```python
from build123d import *

# Parameters (mm, degrees)
SKETCH_1_R      = 7.5
SKETCH_1_R_2    = 2.7
EXTRUDE_1_DEPTH = 3
SKETCH_3_R      = 4
SKETCH_3_R_2    = 2.7
EXTRUDE_3_DEPTH = 32.5
EXTRUDE_START   = -32.5
SKETCH_4_R      = 6
SKETCH_4_R_2    = 2.7
EXTRUDE_4_DEPTH = 32.5


with BuildPart() as part:
    # 草圖1 → 填料-伸長1 (new body)
    with BuildSketch(Plane(origin=(0, 0, 0), x_dir=(1, 0, 0), z_dir=(0, 1, 0))):
        with Locations(Location((0, 0, 0), (0, 0, 270))):
            Circle(SKETCH_1_R)
        with Locations(Location((0, 0, 0), (0, 0, 270))):
            Circle(SKETCH_1_R_2, mode=Mode.SUBTRACT)
    extrude(amount=EXTRUDE_1_DEPTH)

    # 草圖3 → 填料-伸長3 (add)
    with BuildSketch(Plane(origin=(0, 3, 0), x_dir=(1, 0, 0), z_dir=(0, 1, 0))):
        with Locations(Location((0, 0, 0), (0, 0, 270))):
            Circle(SKETCH_3_R)
        with Locations(Location((0, 0, 0), (0, 0, 270))):
            Circle(SKETCH_3_R_2, mode=Mode.SUBTRACT)
    extrude(amount=EXTRUDE_3_DEPTH)

    # 草圖4 → 填料-伸長4 (add)
    with BuildSketch(Plane(origin=(0, 35.5, 0), x_dir=(1, 0, 0), z_dir=(0, 1, 0)).offset(EXTRUDE_START)):
        with Locations(Location((0, 0, 0), (0, 0, 270))):
            Circle(SKETCH_4_R)
        with Locations(Location((0, 0, 0), (0, 0, 270))):
            Circle(SKETCH_4_R_2, mode=Mode.SUBTRACT)
    extrude(amount=EXTRUDE_4_DEPTH)


solid = part.part
```
Geometry: final body of the model. Coordinates: model frame, mm. A direction names the side the tool comes from. Give positions to 0.01 mm unless a question says otherwise; leave off trailing zeros. Loops run counter-clockwise (first coordinate to the right, second up) from the corner with the lowest first, then second, coordinate; pieces in that order, holes last. Notation, with made-up numbers: (60, -9) -> (88, -9) arc R24 ccw to (88, 10) -> close; hole circle Ø5 at (7.25, 81.5). An arc over 180 degrees is marked (long way). Use one line per item in the form item = value.
Item 1: Section query A-A on x = 0. Output: boundary loops of the cut face in (y, z), and give its area (3 significant figures).
A:
outline = (0, -7.5) -> (3, -7.5) -> (3, -6) -> (35.5, -6) -> (35.5, -2.7) -> (0, -2.7) -> close; (0, 2.7) -> (35.5, 2.7) -> (35.5, 6) -> (3, 6) -> (3, 7.5) -> (0, 7.5) -> close
area = 243 mm^2
Item 2: Section query B-B on z = 0. Output: boundary loops of the cut face in (x, y), and give its area (3 significant figures).
A:
outline = (-7.5, 0) -> (-2.7, 0) -> (-2.7, 35.5) -> (-6, 35.5) -> (-6, 3) -> (-7.5, 3) -> close; (2.7, 0) -> (7.5, 0) -> (7.5, 3) -> (6, 3) -> (6, 35.5) -> (2.7, 35.5) -> close
area = 243 mm^2
Item 3: Access query for faces 1 (the face through (6, 3, 2)), 2 (the face through (0.33, 1.479, -7.493)). Directions: +Z, -Z, +X, -X, +Y, -Y. A direction counts if a zero-diameter tool reaches every point of the face in a straight line with its end or side. Return the directions, or none.
A:
face_1 = +Y
face_2 = +Y, -Y
Item 4: Section query C-C on y = 6. Output: boundary loops of the cut face in (x, z), and give its area (3 significant figures).
A:
outline = circle Ø12 at (0, 0); hole circle Ø5.4 at (0, 0)
area = 90.2 mm^2
Item 5: Line query: probe 1 along X at (y, z) = (10, 0); probe 2 along X at (y, z) = (26, -1.25); probe 3 along Z at (x, y) = (2, 13). Output: solid intervals per line, ascending.
A:
probe_1 = -6 to -2.7, 2.7 to 6
probe_2 = -5.87 to -2.39, 2.39 to 5.87
probe_3 = -5.66 to -1.81, 1.81 to 5.66
Item 6: Section query D-D on z = 4.75. Output: boundary loops of the cut face in (x, y), and give its area (3 significant figures).
A:
outline = (-5.8, 0) -> (5.8, 0) -> (5.8, 3) -> (3.67, 3) -> (3.67, 35.5) -> (-3.67, 35.5) -> (-3.67, 3) -> (-5.8, 3) -> close
area = 273 mm^2
Item 7: Pin query (flat end, axial travel): P1, Ø1, axis at x = 3, y = 18, coming from the -Z side; P2, Ø5, axis at x = 6, y = 10, coming from the +Z side; P3, Ø1, axis at x = 0.5, y = 4.5, coming from the +Z side. Return the tip coordinate at first contact, or that it passes through.
A:
P1 = -5.45
P2 = 4.87
P3 = 6
Item 8: Draft query along X for faces 3 (the face through (1.802, 19.022, 5.723)), 4 (the face through (0.811, 17.502, 2.575)), 5 (the face through (0, 0, 3)). Return one class per face: pulls with the +X half, pulls with the -X half, needs draft (parallel to the pull), parting line crosses it, or undercut.
A:
face_3 = parting line crosses it
face_4 = undercut
face_5 = needs draft
